Source: CAD feature listing. Evaluate the final solid. Frame: model axes, mm. A direction names the side the tool comes from. Give positions to 0.01 mm unless a question says otherwise; leave off trailing zeros. Write each loop counter-clockwise with the first axis right and the second up, starting at its lowest first coordinate (ties: lowest second). Pieces come first, ordered by that corner, then holes. Notation, with made-up numbers: (37, -22.5) - (69, -22.5) arc R14 cw to (69, -7.5) - close; hole circle Ø5 at (-34.75, 60). An arc over 180 degrees is marked (long way). Answer as a JSON object with one key per item and string values. Group by question number.
from build123d import *

# Parameters (mm, degrees)
F0_R           = 15.5
F0_R_2         = 13.5
F1_DEPTH       = 15
F2_R           = 27.5
F2_R_2         = 13.5
F3_DEPTH       = 2
F4_R           = 15.5
F4_R_2         = 7.75
F5_DEPTH       = 2
F7_D           = 3.5
F7_CSINK_D     = 6
F7_CSINK_ANGLE = 90


with BuildPart() as f1:
    # F0 (on Top) → F1 (new body)
    with BuildSketch(Plane.XY):
        Circle(F0_R)
        Circle(F0_R_2, mode=Mode.SUBTRACT)
    extrude(amount=-F1_DEPTH)

    # F2 (on Top) → F3 (join)
    with BuildSketch(Plane.XY):
        Circle(F2_R)
        Circle(F2_R_2, mode=Mode.SUBTRACT)
    extrude(amount=F3_DEPTH)

    # F4 (on face) → F5 (join)
    with BuildSketch(Plane(origin=(0, 0, -15), x_dir=(1, 0, 0), z_dir=(0, 0, -1))):
        Circle(F4_R)
        Circle(F4_R_2, mode=Mode.SUBTRACT)
    extrude(amount=F5_DEPTH)

    # F7 (through all)
    with Locations(Plane.XY.offset(2)):
        with Locations((0, 22.5), (-19.485572, -11.25), (19.485572, -11.25)):
            CounterSinkHole(F7_D / 2, F7_CSINK_D / 2, counter_sink_angle=F7_CSINK_ANGLE)


solid = f1.part
Q1. First-contact query: pin 1 Ø4 at (x, y) = (-19.49, -11.25) entering from -Z; pin 2 Ø8 at (x, z) = (-15.5, -13) entering from -Y; pin 3 Ø6 at (y, z) = (-13, -5.5) entering from -X. Flat tips, straight axial feed; report the tip coordinate or a pass-through.
Q2. Section C-C on z = -7. Return the cut outline in (x, y), then the cut area to 3 significant figures.
Q3. Draft query along Y for faces 4 (the cylindrical face through (-21.155, -10.724, 0.37)), 5 (the cylindrical face through (-2.018, -15.368, -8.381)), 6 (the flat face through (-13, -6, 2)). Return one class per face: released by +Y, released by -Y, zero draft, split by the parting line, or undercut.
Q4. Section B-B on y = 3. Return the cut outline in (x, z).
Q5. Ray query, probe 1 along Y at (x, z) = (0, -6); probe 2 along X at (y, z) = (-11.25, 0.5); probe 3 along X at (y, z) = (0, -15.65). Return the intervals inside material, ascending. Write a range as [from, to].
Q6. Section A-A on x = 0. Return the cut outline in (y, z), then the cut area to 3 significant figures.
Q7. Section D-D on y = -11.25. Return the cut outline in (x, z).
Q8. Reachability of faces 1 (the flat face through (6, 6, -15)), 2 (the flat face through (12, -12, 0)), 3 (the cylindrical face through (17.816, -10.724, 0.37)) from +Z, -Z, +X, -X, +Y, -Y: full face, straight path, thin tool, end or side. Return the list, or none.
Taken from the geometry:
{
 "1": {"pin 1": "stops at z = 0", "pin 2": "stops at y = -10.39", "pin 3": "stops at x = -11.84"},
 "2": {"outline": "circle Ø31 at (0, 0); hole circle Ø27 at (0, 0)", "area": "182 mm²"},
 "3": {"face 4": "undercut", "face 5": "split by the parting line", "face 6": "zero draft"},
 "4": {"outline": "(-27.34, 0) - (-15.21, 0) - (-15.21, -17) - (-7.15, -17) - (-7.15, -15) - (-13.16, -15) - (-13.16, 2) - (-27.34, 2) - close; (7.15, -17) - (15.21, -17) - (15.21, 0) - (27.34, 0) - (27.34, 2) - (13.16, 2) - (13.16, -15) - (7.15, -15) - close"},
 "5": {"probe 1": "y = [-15.5, -13.5], [13.5, 15.5]", "probe 2": "x = [-25.09, -21.24], [-17.74, -7.46], [7.46, 17.74], [21.24, 25.09]", "probe 3": "x = [-15.5, -7.75], [7.75, 15.5]"},
 "6": {"outline": "(-27.5, 0) - (-15.5, 0) - (-15.5, -17) - (-7.75, -17) - (-7.75, -15) - (-13.5, -15) - (-13.5, 2) - (-27.5, 2) - close; (7.75, -17) - (15.5, -17) - (15.5, 0) - (20.75, 0) - (20.75, 0.75) - (19.5, 2) - (13.5, 2) - (13.5, -15) - (7.75, -15) - close; (24.25, 0) - (27.5, 0) - (27.5, 2) - (25.5, 2) - (24.25, 0.75) - close", "area": "138 mm²"},
 "7": {"outline": "(-25.09, 0) - (-21.24, 0) - (-21.24, 0.75) - (-22.49, 2) - (-25.09, 2) - close; (-17.74, 0) - (-10.66, 0) - (-10.66, -17) - (10.66, -17) - (10.66, 0) - (17.74, 0) - (17.74, 0.75) - (16.49, 2) - (7.46, 2) - (7.46, -15) - (-7.46, -15) - (-7.46, 2) - (-16.49, 2) - (-17.74, 0.75) - close; (21.24, 0) - (25.09, 0) - (25.09, 2) - (22.49, 2) - (21.24, 0.75) - close"},
 "8": {"face 1": "+Z", "face 2": "-Z", "face 3": "+Z, -Z"}
}
